Source: CAD feature listing. Evaluate the final solid. Frame: model axes, mm. Face numbers are marked on the shaded views. A direction names the side the tool comes from. Give positions to 0.01 mm unless a question says otherwise; leave off trailing zeros. Write each loop counter-clockwise with the first axis right and the second up, starting at its lowest first coordinate (ties: lowest second). Pieces come first, ordered by that corner, then holes. Notation, with made-up numbers: (-33.75, -33.75) -> (-23.75, -33.75) arc R16 cw to (-23.75, -10.75) -> close; hole circle Ø6 at (70.25, 12.5). An arc over 180 degrees is marked (long way). Answer as a JSON object with one key per item and string values. Group by question number.
Item 1: Access query for the marked faces 1, 2 and 3. Directions: +Z, -Z, +X, -X, +Y, -Y. A direction counts if a zero-diameter tool reaches every point of the face in a straight line with its end or side. Return the directions, or none.
Item 2: Section query C-C on y = -9.75. Return the cut outline in (x, z).
Item 3: Ray query, probe 1 along Z at (x, y) = (30.5, -11); probe 2 along Z at (x, y) = (-35, -8); probe 3 along X at (y, z) = (-4.5, 21). Return the intervals inside material, ascending. Write a range as from..to.
Item 4: Pull-direction query (X, two-part tool) for the marked faces 4, 5 and 6; classes: pulls with the +X half, pulls with the -X half, needs draft (parallel to the pull), parting line crosses it, or undercut.
Item 5: Section query D-D on x = -58. Return the cut outline in (y, z), plus the area to 3 significant figures.
Item 6: Section query B-B on x = 2. Return the cut outline in (y, z).
Item 7: Section query A-A on z = 2. Return the cut outline in (x, y), plus the area to 3 significant figures.
Item 8: First-contact query: pin 1 Ø8 at (x, y) = (-15.5, -15) entering from +Z; pin 2 Ø6 at (y, z) = (-9.5, -9.5) entering from +X; pin 3 Ø1.5 at (y, z) = (-12.5, -40) entering from -X. Flat tips, straight axial feed; report the tip coordinate or a pass-through.
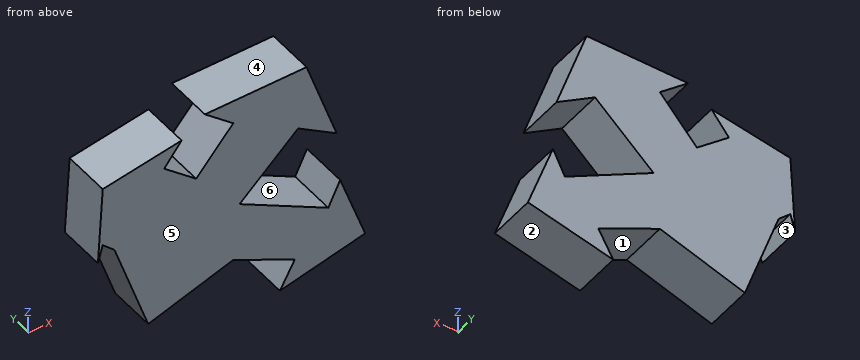
from build123d import *

# Parameters (mm, degrees)
F1_DEPTH = 25.4


with BuildPart() as f1:
    # F0 (on Front) → F1 (new body)
    with BuildSketch(Plane.XZ):
        Polygon((-22.192558, 23.749927), (0, 0), (29.912299, 27.950841), (49.64124, 16.54708), (34.25918, 59.484117), (-17.715111, 56.844085), (-3.21496, 45.55314), align=None)
        Polygon((-51.003944, -8.176205), (-22.192558, 23.749927), (-38.5332, 36.474021), (-29.61387, 47.928478), (-69.954226, 39.32365), (-72.417811, 0), (-69.954226, 8.732829), (-63.947109, 3.504212), align=None)
        Polygon((-24.917955, -24.528613), (0, 0), (-22.192558, 23.749927), (-51.003944, -8.176205), (-63.947109, 3.504212), (-46.721168, -44.579782), (-3.21496, -28.993818), align=None)
        Polygon((45.358468, -22.192556), (0, 0), (-24.917955, -24.528613), (-3.21496, -28.993818), (28.227372, -42.827737), (20.635184, -56.454744), (64.241603, -44.579782), (51.440848, -9.761026), align=None)
    extrude(amount=F1_DEPTH)


solid = f1.part
Worked answers:
{
 "1": {"face 1": "+Y, -Y", "face 2": "-Z, +X, +Y, -Y", "face 3": "-Z, +Y, -Y"},
 "2": {"outline": "(-72.42, 0) -> (-69.95, 8.73) -> (-63.95, 3.5) -> (-46.72, -44.58) -> (-3.21, -28.99) -> (28.23, -42.83) -> (20.64, -56.45) -> (64.24, -44.58) -> (51.44, -9.76) -> (45.36, -22.19) -> (0, 0) -> (29.91, 27.95) -> (49.64, 16.55) -> (34.26, 59.48) -> (-17.72, 56.84) -> (-3.21, 45.55) -> (-22.19, 23.75) -> (-38.53, 36.47) -> (-29.61, 47.93) -> (-69.95, 39.32) -> close"},
 "3": {"probe 1": "-53.77..-14.92, 27.61..59.29", "probe 2": "-40.38..33.72, 41.01..46.78", "probe 3": "-71.1..22.47, 41.94..48.05"},
 "4": {"face 4": "pulls with the -X half", "face 5": "needs draft", "face 6": "undercut"},
 "5": {"outline": "(-25.4, -13.1) -> (0, -13.1) -> (0, 41.87) -> (-25.4, 41.87) -> close", "area": "1,400 mm^2"},
 "6": {"outline": "(-25.4, -31.29) -> (0, -31.29) -> (0, -0.98) -> (-25.4, -0.98) -> close; (-25.4, 1.87) -> (0, 1.87) -> (0, 57.85) -> (-25.4, 57.85) -> close"},
 "7": {"outline": "(-72.29, -25.4) -> (-71.85, -25.4) -> (-71.85, 0) -> (-72.29, 0) -> close; (-63.41, -25.4) -> (2.14, -25.4) -> (2.14, 0) -> (-63.41, 0) -> close", "area": "1,680 mm^2"},
 "8": {"pin 1": "z = 57.16", "pin 2": "x = 52.45", "pin 3": "x = -48.63"}
}
